The listing builds one solid part. Answer for the finished solid, in the listing's coordinates (mm). Coordinates: 2 decimals unless noted, no trailing zeros. Loops run counter-clockwise (first coordinate to the right, second up) from the corner with the lowest first, then second, coordinate; pieces in that order, holes last. Notation, with made-up numbers: (-34, 27) - (15, 27) arc R16 ccw to (15, 36) - close; hole circle Ø10 at (82.5, -20). An arc over 180 degrees is marked (long way). Put each result on its own line as item: value.
```python
from build123d import *

# Parameters (mm, degrees)
F0_R     = 3
F1_DEPTH = 5


with BuildPart() as f1:
    # F0 (on Front) → F1 (new body)
    with BuildSketch(Plane.XZ):
        Polygon((-145, -10), (145, -10), (145, 10), (140, 10), (140, 0), (134.5, 0), (134.5, 10), (129.5, 10), (129.5, 0), (-129.5, 0), (-129.5, 10), (-134.5, 10), (-134.5, 0), (-140, 0), (-140, 10), (-145, 10), align=None)
        with Locations((-137.5, -5)):
            Circle(F0_R, mode=Mode.SUBTRACT)
    extrude(amount=F1_DEPTH)


solid = f1.part
```
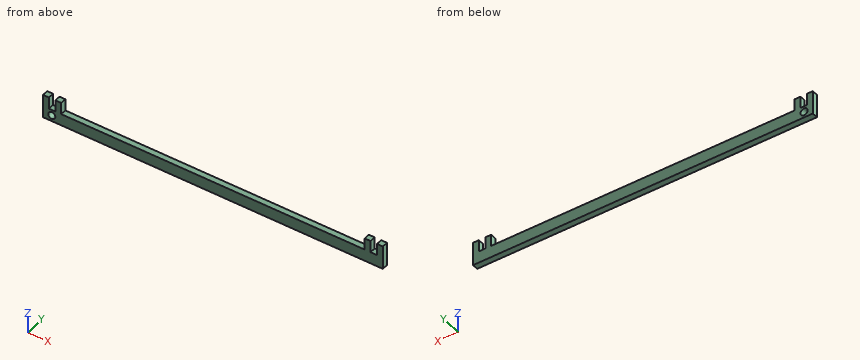
1) The part is cut by section D-D (z = -5). Give the vertices of the cut face in (x, y).
Found:
outline: (-145, -5) - (-140.5, -5) - (-140.5, 0) - (-145, 0) - close; (-134.5, -5) - (145, -5) - (145, 0) - (-134.5, 0) - close
2) Each of these flat-tipped pins is pushed along its axis until it touches: pin 1 (4 mm diameter, centred on x = 25, z = 2.5, fed in from -Y); pin 2 (1.5 mm diameter, centred on x = -138, y = -3.5, fed in from +Z); pin 3 (4 mm diameter, centred on x = 26.5, z = -1.5, fed in from +Y). Where does it stop, or does it pass through?
Found:
pin 1: passes through
pin 2: stops at z = 0
pin 3: stops at y = 0
3) The part is cut by section A-A (z = 5.75). Give the vertices of the cut face in (x, y), and give its area (3 significant figures).
Found:
outline: (-145, -5) - (-140, -5) - (-140, 0) - (-145, 0) - close; (-134.5, -5) - (-129.5, -5) - (-129.5, 0) - (-134.5, 0) - close; (129.5, -5) - (134.5, -5) - (134.5, 0) - (129.5, 0) - close; (140, -5) - (145, -5) - (145, 0) - (140, 0) - close
area: 100 mm^2
4) Straight lines are drawn through the part: L1, parallel to X at y = -0.6, z = 6.25; L2, parallel to Z at x = -137.5, y = -2.75; L3, parallel to Z at x = 42, y = -0.75. For each, find the intervals that lie inside material, in ascending order. Write a range as [from, to].
Found:
L1: x = [-145, -140], [-134.5, -129.5], [129.5, 134.5], [140, 145]
L2: z = [-10, -8], [-2, 0]
L3: z = [-10, 0]
5) The part is cut by section C-C (y = -1.1). Give the vertices of the cut face in (x, z).
Found:
outline: (-145, -10) - (145, -10) - (145, 10) - (140, 10) - (140, 0) - (134.5, 0) - (134.5, 10) - (129.5, 10) - (129.5, 0) - (-129.5, 0) - (-129.5, 10) - (-134.5, 10) - (-134.5, 0) - (-140, 0) - (-140, 10) - (-145, 10) - close; hole circle Ø6 at (-137.5, -5)
6) The part is cut by section B-B (x = -137.5). Give the vertices of the cut face in (y, z), and give its area (3 significant figures).
Found:
outline: (-5, -10) - (0, -10) - (0, -8) - (-5, -8) - close; (-5, -2) - (0, -2) - (0, 0) - (-5, 0) - close
area: 20.0 mm^2
